```python
from build123d import *

# Parameters (mm, degrees)
F0_R     = 51
F1_DEPTH = 1800
F2_R     = 90
F3_DEPTH = 100
F4_R     = 38
F5_DEPTH = 200.001


with BuildPart() as f1:
    # F0 (on Top) → F1 (new body)
    with BuildSketch(Plane.XY):
        Circle(F0_R)
    extrude(amount=F1_DEPTH)

    # F2 (on Right) → F3 (join, symmetric)
    with BuildSketch(Plane.YZ):
        with Locations((0, 1800)):
            Circle(F2_R)
    extrude(amount=F3_DEPTH, both=True)

    # F4 (on face) → F5 (cut, through all)
    with BuildSketch(Plane.YZ.offset(100)):
        with Locations((0, 1800)):
            Circle(F4_R)
    extrude(amount=-F5_DEPTH, mode=Mode.SUBTRACT)


solid = f1.part
```
The model under review builds one solid part; all positions refer to its coordinate system, in mm. Round coordinates to 2 decimals unless told otherwise and drop trailing zeros. Loops run counter-clockwise (first coordinate to the right, second up) from the corner with the lowest first, then second, coordinate; pieces in that order, holes last. Notation, with made-up numbers: (47, -10.5) -> (70, -10.5) arc R15 ccw to (70, 1.5) -> close; hole circle Ø9 at (30, -30.75). An arc over 180 degrees is marked (long way). Answer in a Markdown table with one row per item.
1) Consider section A-A, the plane y = 0. Write out the cut boundary in (x, z).
Taken from the geometry:
| item | result |
|---|---|
| outline | (-100, 1710) -> (-51, 1710) -> (-51, 0) -> (51, 0) -> (51, 1710) -> (100, 1710) -> (100, 1762) -> (-100, 1762) -> close; (-100, 1838) -> (100, 1838) -> (100, 1890) -> (-100, 1890) -> close |
2) Consider section B-B, the plane x = 0. Write out the cut boundary in (y, z).
Taken from the geometry:
| item | result |
|---|---|
| outline | (-51, 0) -> (51, 0) -> (51, 1725.84) arc R90 ccw (long way) to (-51, 1725.84) -> close; hole circle Ø76 at (0, 1800) |
3) Consider section D-D, the plane x = 72. Write out the cut boundary in (y, z).
Taken from the geometry:
| item | result |
|---|---|
| outline | circle Ø180 at (0, 1800); hole circle Ø76 at (0, 1800) |
4) Draft analysis for pull direction Z (two halves, no side actions). For faces 1 (the cylindrical face through (-11.056, -49.787, 850.841)), 2 (the cylindrical face through (1.4, -4.947, 1837.677)), 3 (the cylindrical face through (1.4, -11.716, 1889.234)), state which applies: pulls with the +Z half, pulls with the -Z half, needs draft (parallel to the pull), parting line crosses it, or undercut.
Taken from the geometry:
| item | result |
|---|---|
| face 1 | needs draft |
| face 2 | undercut |
| face 3 | parting line crosses it |
5) Wall thickness on line 1 along Z through (x, y) = (59.5, 0); line 2 along Z through (x, y) = (19, 0); line 3 along X through (y, z) = (-3, 1459.5): over which ranges is each line inside the solid? List them lowest first.
Taken from the geometry:
| item | result |
|---|---|
| line 1 | z = 1710 to 1762, 1838 to 1890 |
| line 2 | z = 0 to 1762, 1838 to 1890 |
| line 3 | x = -50.91 to 50.91 |
6) Consider section C-C, the plane z = 1097.5. Write out the cut boundary in (x, y).
Taken from the geometry:
| item | result |
|---|---|
| outline | circle Ø102 at (0, 0) |
7) For pin 1 Ø2 at (y, z) = (28.5, 627) entering from +X; pin 2 Ø5 at (x, y) = (54.5, -19) entering from +Z; pin 3 Ø2 at (x, z) = (-45, 590.5) entering from +Y, all flat-tipped, find the tip position at first contact; note any pin that passes through.
Taken from the geometry:
| item | result |
|---|---|
| pin 1 | stops at x = 42.95 |
| pin 2 | stops at z = 1888.47 |
| pin 3 | stops at y = 25.79 |
